from build123d import *

# Parameters (mm, degrees)
F0_W     = 38.2953844965
F0_H     = 31.7133665085
F1_DEPTH = 25.4
F2_W     = 38.2953844965
F2_H     = 18.9767321572
F3_DEPTH = 12.7
F5_DEPTH = 12.701


with BuildPart() as f1:
    # F0 (on Front) → F1 (new body)
    with BuildSketch(Plane.XZ):
        with Locations((19.1476922482, 15.8566832542)):
            Rectangle(F0_W, F0_H)
    extrude(amount=F1_DEPTH)

    # F2 (on face) → F3 (cut)
    with BuildSketch(Plane.XZ.offset(25.4)):
        with Locations((19.1476922482, 22.2250004299)):
            Rectangle(F2_W, F2_H)
    extrude(amount=-F3_DEPTH, mode=Mode.SUBTRACT)

    # F4 (on face) → F5 (cut, through all)
    with BuildSketch(Plane.XZ.offset(12.7)):
        Polygon((38.2953844965, 31.7133665085), (25.4732687026, 31.7133665085), (38.2953844965, 12.7366343513), align=None)
    extrude(amount=-F5_DEPTH, mode=Mode.SUBTRACT)


solid = f1.part
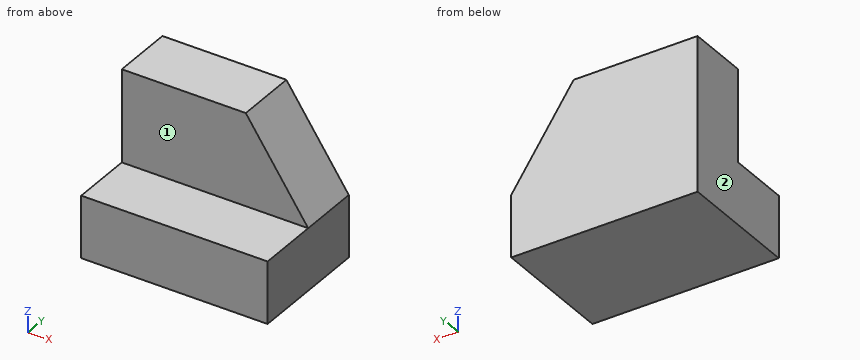
Model file for the job. Use its own axes, mm. Face numbers are marked on the shaded views. A direction names the side the tool comes from. Coordinates: 2 decimals unless noted, no trailing zeros. Order: outer loops, then holes, each group sorted by start corner. A loop starts at its lowest first (then second) coordinate and runs counter-clockwise, first axis right, second up. Notation, with made-up numbers: M -27,7.25 L 1,7.25 A28 cw 1,31.25 Z; hole C -18.75,28.5 d6. An arc over 180 degrees is marked long. Return JSON: item names as keys, results as strings.
1. Flat gauge pins, fed straight in: pin 1 (2 mm diameter, centred on x = 29.5, y = -16.5, fed in from +Z); pin 2 (1.5 mm diameter, centred on x = 24.5, z = 14.5, fed in from -Y); pin 3 (10 mm diameter, centred on y = -5, z = 18, fed in from +X). Where does each tip first touch, or does it go through?
Ans:
{"pin 1": "z = 12.74", "pin 2": "y = -12.7", "pin 3": "x = 38.12"}
2. Drill centre lines: probe 1 along Z at (x, y) = (16, -14.75); probe 2 along Y at (x, z) = (9, 20.5); probe 3 along X at (y, z) = (-12, 30). Where is each one in solid material? Low to high.
Ans:
{"probe 1": "0 to 12.74", "probe 2": "-12.7 to 0", "probe 3": "0 to 26.63"}
3. Saw through at B-B (x = 5). Give the cut face in (y, z), and give its area (3 significant figures).
Ans:
{"outline": "M -25.4,0 L 0,0 L 0,31.71 L -12.7,31.71 L -12.7,12.74 L -25.4,12.74 Z", "area": "565 mm^2"}
4. Saw through at A-A (y = -8). Give the cut face in (x, z).
Ans:
{"outline": "M 0,0 L 38.3,0 L 38.3,12.74 L 25.47,31.71 L 0,31.71 Z"}
5. Saw through at D-D (y = -16.5). Give the cut face in (x, z), and give its area (3 significant figures).
Ans:
{"outline": "M 0,0 L 38.3,0 L 38.3,12.74 L 0,12.74 Z", "area": "488 mm^2"}
6. Saw through at C-C (z = 23.5). Give the cut face in (x, y).
Ans:
{"outline": "M 0,-12.7 L 31.02,-12.7 L 31.02,0 L 0,0 Z"}
7. Tool access for the marked faces 1 and 2: list every direction of +Z, -Z, +X, -X, +Y, -Y with a clear straight run to the whole face (end or side of a thin tool).
Ans:
{"face 1": "+Z, +X, -X, -Y", "face 2": "+Z, -Z, -X, +Y, -Y"}
